Geometry: see drawing. Coordinates: mm, zero at the bounding-box minimum. A direction names the side the tool comes from. Round coordinates to 2 decimals unless told otherwise and drop trailing zeros. Order: outer loops, then holes, each group sorted by start corner. A loop starts at its lowest first (then second) coordinate and runs counter-clockwise, first axis right, second up.
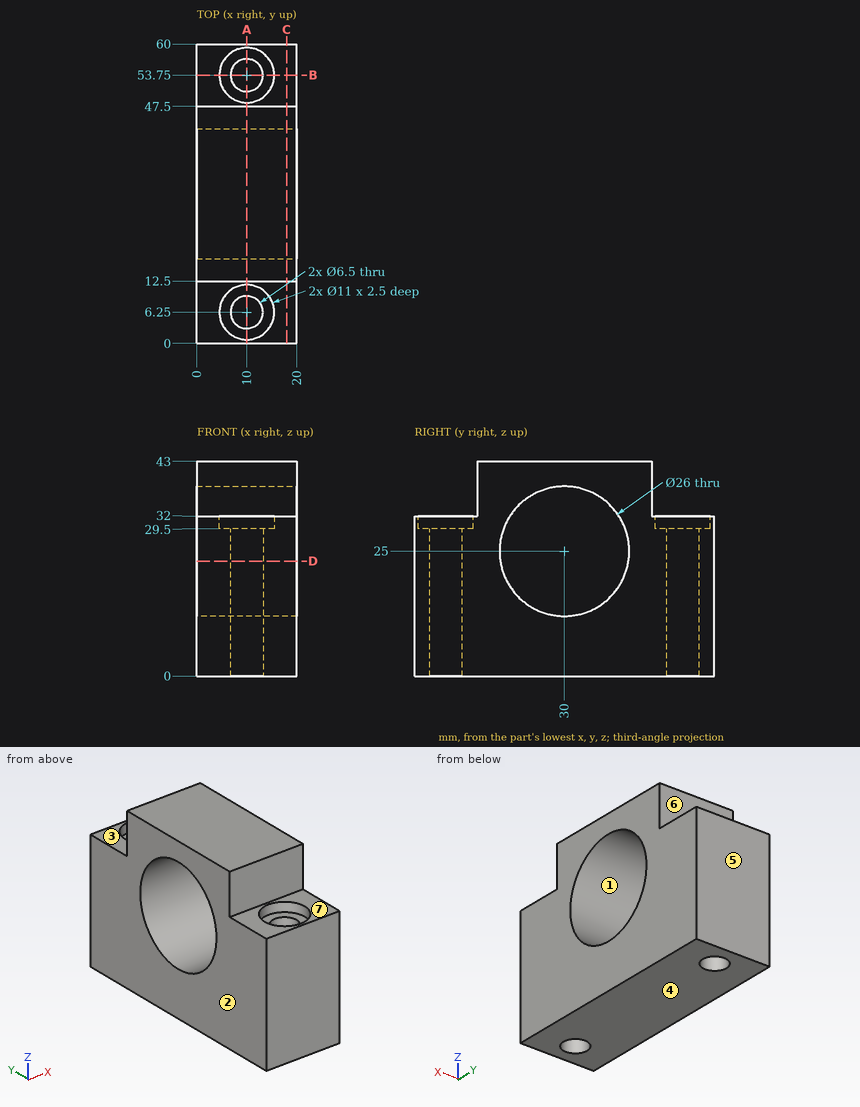
1. Line query: line 1 along Y through (x, z) = (8.5, 29); line 2 along Y through (x, z) = (9.5, 8); line 3 along Y through (x, z) = (12, 22.5). Output: solid intervals per line, ascending.
2. Section C-C on x = 18. Return loops of the section in (y, z), plus the area to 3 significant figures.
3. Access query for the marked faces 5, 6 and 7. Directions: +Z, -Z, +X, -X, +Y, -Y. A direction counts if a zero-diameter tool reaches every point of the face in a straight line with its end or side. Return the directions, or none.
4. Pull-direction query (Z, two-part tool) for the marked faces 1, 2, 3 and 4; classes: released by +Z, released by -Z, zero draft, split by the parting line, or undercut.
5. Section A-A on x = 10. Return loops of the section in (y, z), plus the area to 3 significant figures.
6. First-contact query: pin 1 (7.5 mm diameter, centred on x = 10, y = 6.25, fed in from +Z); pin 2 (12 mm diameter, centred on x = 12.5, y = 54.5, fed in from +Z); pin 3 (4 mm diameter, centred on x = 11, z = 31.5, fed in from -Y); pin 4 (12 mm diameter, centred on x = 12.5, z = 39.5, fed in from -Y). Flat tips, straight axial feed; report the tip coordinate or a pass-through.
7. Section D-D on z = 23. Return loops of the section in (x, y).
8. Section B-B on y = 53.75. Return loops of the section in (x, z).
Result:
1. line 1: y = 0 to 3.37, 9.13 to 17.63, 42.37 to 50.87, 56.63 to 60
1. line 2: y = 0 to 3.04, 9.46 to 50.54, 56.96 to 60
1. line 3: y = 0 to 3.69, 8.81 to 17.24, 42.76 to 51.19, 56.31 to 60
2. outline: (0, 0) - (60, 0) - (60, 32) - (47.5, 32) - (47.5, 43) - (12.5, 43) - (12.5, 32) - (0, 32) - close; hole circle Ø26 at (30, 25)
2. area: 1,770 mm2
3. face 5: +Z, -Z, +X, -X, +Y
3. face 6: +Z, +X, -X, +Y
3. face 7: +Z, +X, -X, -Y
4. face 1: undercut
4. face 2: zero draft
4. face 3: released by +Z
4. face 4: released by -Z
5. outline: (0, 0) - (3, 0) - (3, 29.5) - (0.75, 29.5) - (0.75, 32) - (0, 32) - close; (9.5, 0) - (50.5, 0) - (50.5, 29.5) - (48.25, 29.5) - (48.25, 32) - (47.5, 32) - (47.5, 43) - (12.5, 43) - (12.5, 32) - (11.75, 32) - (11.75, 29.5) - (9.5, 29.5) - close; (57, 0) - (60, 0) - (60, 32) - (59.25, 32) - (59.25, 29.5) - (57, 29.5) - close; hole circle Ø26 at (30, 25)
5. area: 1,340 mm2
6. pin 1: stops at z = 29.5
6. pin 2: stops at z = 32
6. pin 3: stops at y = 0
6. pin 4: stops at y = 12.5
7. outline: (0, 0) - (20, 0) - (20, 17.15) - (0, 17.15) - close; (0, 42.85) - (20, 42.85) - (20, 60) - (0, 60) - close; hole circle Ø6.5 at (10, 6.25); hole circle Ø6.5 at (10, 53.75)
8. outline: (0, 0) - (6.75, 0) - (6.75, 29.5) - (4.5, 29.5) - (4.5, 32) - (0, 32) - close; (13.25, 0) - (20, 0) - (20, 32) - (15.5, 32) - (15.5, 29.5) - (13.25, 29.5) - close
